Build history of the part. All positions in model axes, mm. A direction names the side the tool comes from. Coordinates: 2 decimals unless noted, no trailing zeros. Loops run counter-clockwise (first coordinate to the right, second up) from the corner with the lowest first, then second, coordinate; pieces in that order, holes last. Notation, with made-up numbers: (-35, 34) - (-9, 34) arc R30 ccw to (-9, 64) - close; hole circle Ø9 at (75.25, 29.25). An arc over 180 degrees is marked (long way). One line per item, written item: value.
```python
from build123d import *

# Parameters (mm, degrees)
CHAMFER1_SIZE           = 1
CUT_EXTRUDE1_DEPTH      = 48.370877129
CUT_EXTRUDE1_DEPTH_BACK = 48.370877129
SKETCH2_R               = 5.5


with BuildPart() as part:
    # Sketch1 → Revolve1 (revolve)
    with BuildSketch(Plane(origin=(0, 0, 0), x_dir=(1, 0, 0), z_dir=(0, 1, 0)), mode=Mode.PRIVATE) as revolve1_sk:
        Polygon((17, 4), (0, 4), (0, 8), (10, 8), (10, 25), (6.7, 25), (6.7, 30), (7.4, 30), (7.4, 32), (16.6, 32), (16.6, 30), (17.3, 30), (17.3, 25), (14, 25), (14, 6), (17, 6), align=None)
    revolve(revolve1_sk.sketch.rotate(Axis((0, 0, 0), (1, 0, 0)), 180), axis=Axis((0, 0, 0), (1, 0, 0)))

    # Chamfer1
    chamfer1_edges = [part.edges().sort_by_distance(p)[0] for p in [
        (0, 0, -4),
        (17, 0, -4),
    ]]
    chamfer(chamfer1_edges, length=CHAMFER1_SIZE)

    # Sketch2 → Cut-Extrude1 (cut, two sides: drawn at the far end of the back side and taken through both)
    with BuildSketch(Plane(origin=(14, 0, 0), x_dir=(0, 0, -1), z_dir=(1, 0, 0)).offset(-CUT_EXTRUDE1_DEPTH_BACK)):
        with Locations((-16.5, 0)):
            Circle(SKETCH2_R)
        with Locations((-8.25, 14.289419162)):
            Circle(SKETCH2_R)
        with Locations((8.25, 14.289419162)):
            Circle(SKETCH2_R)
        with Locations((16.5, 0)):
            Circle(SKETCH2_R)
        with Locations((8.25, -14.289419162)):
            Circle(SKETCH2_R)
        with Locations((-8.25, -14.289419162)):
            Circle(SKETCH2_R)
    extrude(amount=CUT_EXTRUDE1_DEPTH + CUT_EXTRUDE1_DEPTH_BACK, mode=Mode.SUBTRACT)


solid = part.part
```
Item 1: Cut at B-B, the plane y = 0. Give the number of separate pieces and of enclosed holes in the cut face, then the cut area to 3 significant figures.
Check result:
separate pieces: 4
enclosed holes: 0
area: 313 mm^2
Item 2: Cut at A-A, the plane z = 16.5. Write the cut outline in (x, y), then the cut area to 3 significant figures.
Check result:
outline: (6.7, -25.05) - (7.4, -25.05) - (7.4, -27.42) - (16.6, -27.42) - (16.6, -25.05) - (17.3, -25.05) - (17.3, -18.78) - (14, -18.78) - (14, -5.5) - (10, -5.5) - (10, -18.78) - (6.7, -18.78) - close; (6.7, 18.78) - (10, 18.78) - (10, 5.5) - (14, 5.5) - (14, 18.78) - (17.3, 18.78) - (17.3, 25.05) - (16.6, 25.05) - (16.6, 27.42) - (7.4, 27.42) - (7.4, 25.05) - (6.7, 25.05) - close
area: 283 mm^2
Item 3: Cut at C-C, the plane x = 5. Write the cut outline in (y, z), then the cut area to 3 significant figures.
Check result:
outline: circle Ø16 at (0, 0); hole circle Ø8 at (0, 0)
area: 151 mm^2
Item 4: Pull direction Z, two halves, no side cores. Call faces 1 (the face through (16.6, 9, -29)), 2 (the face through (7.055, -25.296, 16.128)), 3 (the face through (17, -4, -4)): released by +Z, released by -Z, zero draft, split by the parting line, or undercut.
Check result:
face 1: zero draft
face 2: split by the parting line
face 3: undercut
Item 5: Drop flat-ended pins along their axis: P1, Ø10, axis at y = 0, z = -16.5, coming from the +X side; P2, Ø3, axis at y = 5.5, z = 7.5, coming from the +X side; P3, Ø2, axis at x = 7, y = -14.5, coming from the +Z side; P4, Ø8, axis at x = 14, y = -21, coming from the +Z side. Give the stop position or say it passes through.
Check result:
P1: passes through
P2: stops at x = 14
P3: stops at z = 28.97
P4: stops at z = 27.11
Item 6: Probe probe 1 along Y at (x, z) = (7.65, 0); probe 2 along Y at (x, z) = (6.75, 0); probe 3 along Z at (x, y) = (8.5, 3). List the from-to ranges inside material, lowest first. Write a range as from..to.
Check result:
probe 1: y = -32..-25, -8..-4, 4..8, 25..32
probe 2: y = -30..-25, -8..-4, 4..8, 25..30
probe 3: z = -31.86..-24.82, -7.42..-2.65, 2.65..7.42, 24.82..31.86
Item 7: Tool access for faces 4 (the face through (15.521, -1.802, 5.723)), 5 (the face through (7.4, -29, -9)), 6 (the face through (11.97, -2.11, -21.58)): list every direction of +Z, -Z, +X, -X, +Y, -Y with a clear straight run to the whole face (end or side of a thin tool).
Check result:
face 4: +X
face 5: -X
face 6: +X, -X
Item 8: Cut at D-D, the plane z = 9. Write the cut outline in (x, y).
Check result:
outline: (6.7, -28.62) - (7.4, -28.62) - (7.4, -30.71) - (16.6, -30.71) - (16.6, -28.62) - (17.3, -28.62) - (17.3, -23.32) - (14, -23.32) - (14, -19.74) - (10, -19.74) - (10, -23.32) - (6.7, -23.32) - close; (6.7, 23.32) - (10, 23.32) - (10, 19.74) - (14, 19.74) - (14, 23.32) - (17.3, 23.32) - (17.3, 28.62) - (16.6, 28.62) - (16.6, 30.71) - (7.4, 30.71) - (7.4, 28.62) - (6.7, 28.62) - close; (10, -8.84) - (14, -8.84) - (14, 8.84) - (10, 8.84) - close
